Geometry: final body of the model. Coordinates: model frame, mm. Face numbers are marked on the shaded views. A direction names the side the tool comes from. Give positions to 0.01 mm unless a question says otherwise; leave off trailing zeros. Write each loop counter-clockwise with the first axis right and the second up, starting at its lowest first coordinate (ties: lowest second). Pieces come first, ordered by that corner, then holes. Notation, with made-up numbers: M 16.5,39 L 38.5,39 A23 cw 38.5,56 Z; hole C 83,22 d6. An arc over 180 degrees is marked long. Answer as a JSON object with one key per item and string values.
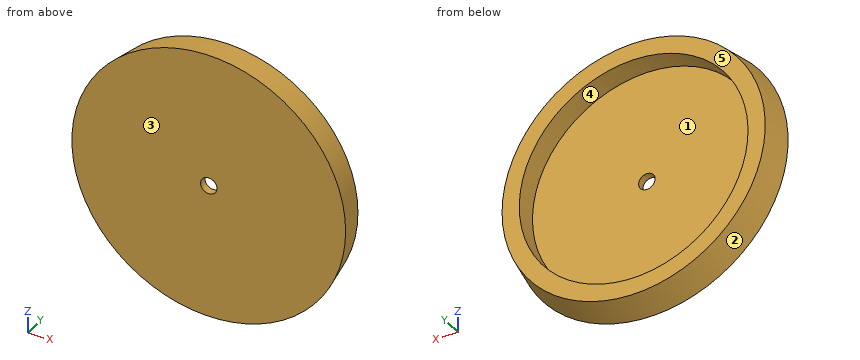
from build123d import *

# Parameters (mm, degrees)
SKETCH1_R           = 18.25
BOSS_EXTRUDE1_DEPTH = 4
BOSS_EXTRUDE1_TAPER = 10
CUT_EXTRUDE2_START  = 4
SKETCH1_5_R         = 1.1
CUT_EXTRUDE2_DEPTH  = 4
CUT_EXTRUDE3_START  = 4
SKETCH1_6_R         = 15.25
CUT_EXTRUDE3_DEPTH  = 3


with BuildPart() as part:
    # Sketch1 → Boss-Extrude1 (new body)
    with BuildSketch(Plane(origin=(0, 0, 0), x_dir=(1, 0, 0), z_dir=(0, 1, 0))):
        Circle(SKETCH1_R)
    extrude(amount=BOSS_EXTRUDE1_DEPTH, taper=BOSS_EXTRUDE1_TAPER)

    # Sketch1<5> → Cut-Extrude2 (cut)
    with BuildSketch(Plane(origin=(0, 0, 0), x_dir=(1, 0, 0), z_dir=(0, 1, 0)).offset(CUT_EXTRUDE2_START)):
        with Locations(Location((0, 0, 0), (0, 0, 270))):
            Circle(SKETCH1_5_R)
    extrude(amount=-CUT_EXTRUDE2_DEPTH, mode=Mode.SUBTRACT)

    # Sketch1<6> → Cut-Extrude3 (cut)
    with BuildSketch(Plane(origin=(0, 0, 0), x_dir=(1, 0, 0), z_dir=(0, 1, 0)).offset(CUT_EXTRUDE3_START)):
        with Locations(Location((0, 0, 0), (0, 0, 270))):
            Circle(SKETCH1_6_R)
    extrude(amount=-CUT_EXTRUDE3_DEPTH, mode=Mode.SUBTRACT)


solid = part.part
1) Pull-direction query (X, two-part tool) for the marked faces 1, 2 and 3; classes: pulls with the +X half, pulls with the -X half, needs draft (parallel to the pull), parting line crosses it, or undercut.
Geometry check:
{"face 1": "undercut", "face 2": "parting line crosses it", "face 3": "needs draft"}
2) Line query: line 1 (Y direction, x = 1, z = 14); line 2 (X direction, y = 0.55, z = 0); line 3 (X direction, y = 1.4, z = 8.5). Output: solid intervals per line, ascending. Write a range as from..to.
Geometry check:
{"line 1": "y = 0..1", "line 2": "x = -18.15..-1.1, 1.1..18.15", "line 3": "x = -15.87..-12.66, 12.66..15.87"}
3) Contact query for flat-ended pins moving along their axis: P1, Ø1.5, axis at y = 3, z = -9, coming from the -X side; P2, Ø2, axis at x = 4.5, y = 3.5, coming from the -Z side; P3, Ø1.5, axis at x = 8.5, z = 6, coming from the +Y side. Output: stop coordinate, or through.
Geometry check:
{"P1": "stops at x = -15.71", "P2": "stops at z = -17.35", "P3": "stops at y = 1"}
4) Cut plane A-A on x = 0. Return loops of the section in (y, z), and give its area (3 significant figures).
Geometry check:
{"outline": "M 0,-18.25 L 4,-17.54 L 4,-15.25 L 1,-15.25 L 1,-1.1 L 0,-1.1 Z; M 0,1.1 L 1,1.1 L 1,15.25 L 4,15.25 L 4,17.54 L 0,18.25 Z", "area": "49.5 mm2"}
5) Cut plane B-B on y = 2.35. Return loops of the section in (x, z), and give its area (3 significant figures).
Geometry check:
{"outline": "C 0,0 d35.67; hole C 0,0 d30.5", "area": "269 mm2"}
6) Set-up query: the marked faces 4 and 5. Return all of +Z, -Z, +X, -X, +Y, -Y with unobstructed straight access to the full face (end or side cutting, diameter ignored); none if empty.
Geometry check:
{"face 4": "+Y", "face 5": "+Z, -Z, +X, -X, +Y"}
